Check sheet for the modelled part. Datum: model origin and axes. Units: mm. Face numbers are marked on the shaded views. A direction names the side the tool comes from. Coordinates: 2 decimals unless noted, no trailing zeros. Order: outer loops, then holes, each group sorted by start corner. A loop starts at its lowest first (then second) coordinate and runs counter-clockwise, first axis right, second up.
1. Thickness scan on line 1 (X direction, y = -74, z = 7); line 2 (Y direction, x = 19.5, z = 8); line 3 (Z direction, x = -51.5, y = -31). Record the ranges inside material, lowest first.
2. Cross-section at A-A (y = 27.5). Enter the section's corners in (x, z), then the cut area to 3 significant figures.
3. Gauge pin test, flat ends, axial feed: pin 1 Ø4 at (x, y) = (-101.5, 59) entering from +Z; pin 2 Ø9 at (x, y) = (-8, -97) entering from +Z. Record the tip position at first contact, or that the pin passes through.
4. Cross-section at C-C (y = 89). Enter the section's corners in (x, z), then the cut area to 3 significant figures.
5. Set-up check for the marked faces 1 and 2: record each of +Z, -Z, +X, -X, +Y, -Y from which the full face is reachable in a straight line by a thin tool's end or side.
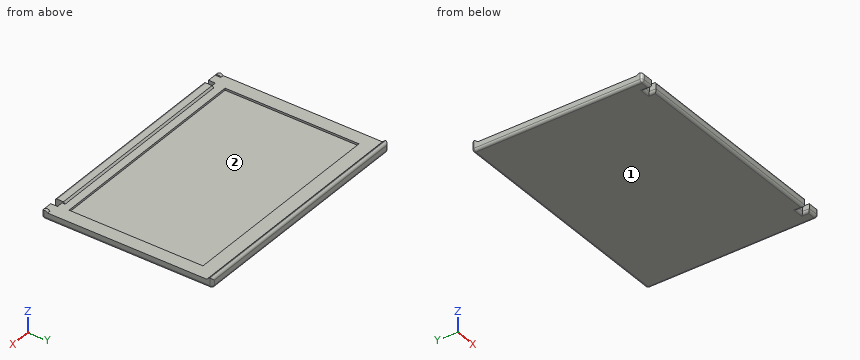
```python
from build123d import *

# Parameters (mm, degrees)
SKETCH1_W           = 295
SKETCH1_H           = 209
BOSS_EXTRUDE1_DEPTH = 9
SKETCH2_W           = 262
SKETCH2_H           = 164
CUT_EXTRUDE1_DEPTH  = 2.5
SKETCH3_W           = 3
SKETCH3_H           = 3
BOSS_EXTRUDE2_DEPTH = 295
CHAMFER1_SIZE       = 4
SKETCH4_W           = 7.7
SKETCH4_H           = 8.3
CUT_EXTRUDE2_DEPTH  = 250
BOSS_EXTRUDE3_DEPTH = 4
SKETCH6_W           = 249.6
SKETCH6_H           = 10
BOSS_EXTRUDE4_DEPTH = 2
CHAMFER2_SIZE       = 2
FILLET1_R           = 2
FILLET2_R           = 3


# Some blends are built 0.0001 mm under size
with BuildPart() as part:
    # Sketch1 → Boss-Extrude1 (new body)
    with BuildSketch(Plane.XY):
        Rectangle(SKETCH1_W, SKETCH1_H)
    extrude(amount=BOSS_EXTRUDE1_DEPTH)

    # Sketch2 → Cut-Extrude1 (cut)
    with BuildSketch(Plane.XY.offset(9)):
        with Locations((0, -1.2)):
            Rectangle(SKETCH2_W, SKETCH2_H)
    extrude(amount=-CUT_EXTRUDE1_DEPTH, mode=Mode.SUBTRACT)

    # Sketch3 → Boss-Extrude2 (add)
    with BuildSketch(Plane(origin=(147.5, 0, 0), x_dir=(0, 0, -1), z_dir=(1, 0, 0))):
        with Locations((-10.5, 103)):
            Rectangle(SKETCH3_W, SKETCH3_H)
    extrude(amount=-BOSS_EXTRUDE2_DEPTH)

    # Chamfer1
    # the kernel refuses this chamfer: 4 mm, written as the material it adds along each edge
    with BuildSketch(Plane(origin=(147.5, 101.5, 9), x_dir=(0, -0.9996219169112968, -0.02749587661058651), z_dir=(-1, 0, 0))) as chamfer1_piece_1_section:
        Polygon((CHAMFER1_SIZE * 0.999621916911, CHAMFER1_SIZE * 0.0274958766106), (-CHAMFER1_SIZE * 0.0274958766106, CHAMFER1_SIZE * 0.999621916911), (0, 0), align=None)
    chamfer1_piece_1 = extrude(amount=295, mode=Mode.PRIVATE)
    chamfer1_piece_1 = split(chamfer1_piece_1, bisect_by=Plane(origin=(0, 100.092163559, 12), z_dir=(0, 0, -1)), keep=Keep.TOP, mode=Mode.PRIVATE)
    add(chamfer1_piece_1)

    # Sketch4 → Cut-Extrude2 (cut)
    with BuildSketch(Plane.XY.offset(9)):
        with Locations((-128.65, -100.35)):
            Rectangle(SKETCH4_W, SKETCH4_H)
        with Locations((128.65, -100.35)):
            Rectangle(SKETCH4_W, SKETCH4_H)
    extrude(amount=-CUT_EXTRUDE2_DEPTH, mode=Mode.SUBTRACT)

    # Sketch5 → Boss-Extrude3 (add)
    with BuildSketch(Plane(origin=(147.5, 0, 0), x_dir=(0, 0, -1), z_dir=(1, 0, 0))):
        with BuildLine():
            Line((-9, -104.5), (-9, -97.5))
            ThreePointArc((-9, -97.5), (-10.671572875, -101), (-9, -104.5))
        make_face()
    boss_extrude3 = extrude(amount=-BOSS_EXTRUDE3_DEPTH)

    # Mirror1: Boss-Extrude3 across plane
    add(boss_extrude3.mirror(Plane(origin=(0, 0, 0), x_dir=(0, 0, 1), z_dir=(1, 0, 0))))

    # Sketch6 → Boss-Extrude4 (add)
    with BuildSketch(Plane.XY.offset(9)):
        with Locations((0, -99.5)):
            Rectangle(SKETCH6_W, SKETCH6_H)
    extrude(amount=BOSS_EXTRUDE4_DEPTH)

    # Chamfer2
    chamfer2_edges = [part.edges().sort_by_distance(p)[0] for p in [
        (0, -94.5, 9),
    ]]
    chamfer(chamfer2_edges, length=CHAMFER2_SIZE - 0.0001)  # a hair under: the kernel refuses the full size

    # Fillet1
    fillet1_edges = [part.edges().sort_by_distance(p)[0] for p in [
        (0, -104.5, 11),
    ]]
    fillet(fillet1_edges, radius=FILLET1_R)

    # Fillet2
    fillet2_edges = [part.edges().sort_by_distance(p)[0] for p in [
        (0, 104.5, 12),
        (0, 104.5, 0),
        (0, -104.5, 0),
        (147.5, 0, 0),
        (-124.8, -100.35, 0),
        (-128.65, -96.2, 0),
        (-132.5, -100.35, 0),
        (-140, -104.5, 0),
        (-147.5, 0, 0),
        (140, -104.5, 0),
        (132.5, -100.35, 0),
        (128.65, -96.2, 0),
        (124.8, -100.35, 0),
        (-147.5, 104.5, 6),
        (147.5, 104.5, 6),
        (147.5, -104.5, 4.5),
        (-147.5, -104.5, 4.5),
    ]]
    fillet(fillet2_edges, radius=FILLET2_R)


solid = part.part
```
Data:
1. line 1: x = -147.5 to -131, 131 to 147.5
1. line 2: y = -104.5 to -83.2, 80.8 to 104.5
1. line 3: z = 0 to 6.5
2. outline: (-147.5, 3) arc R3 ccw to (-144.5, 0) - (144.5, 0) arc R3 ccw to (147.5, 3) - (147.5, 9) - (131, 9) - (131, 6.5) - (-131, 6.5) - (-131, 9) - (-147.5, 9) - close
2. area: 2,000 mm2
3. pin 1: stops at z = 6.5
3. pin 2: stops at z = 11
4. outline: (-147.5, 3) arc R3 ccw to (-144.5, 0) - (144.5, 0) arc R3 ccw to (147.5, 3) - (147.5, 9) - (-147.5, 9) - close
4. area: 2,650 mm2
5. face 1: -Z, +X, -X, +Y, -Y
5. face 2: +Z
